from build123d import *

# Parameters (mm, degrees)
F1_DEPTH = 25.4
F2_T     = -0.254


with BuildPart() as f1:
    # F0 (on Top) → F1 (new body)
    with BuildSketch(Plane.XY):
        with BuildLine():
            Line((-3.175, 0), (0, 0))
            Line((0, 0), (0, 25.4))
            ThreePointArc((0, 25.4), (25.4, 50.8), (50.8, 25.4))
            Line((50.8, 25.4), (50.8, 0))
            Line((50.8, 0), (53.975, 0))
            Line((53.975, 0), (53.975, 25.4))
            ThreePointArc((53.975, 25.4), (25.4, 53.975), (-3.175, 25.4))
            Line((-3.175, 25.4), (-3.175, 0))
        make_face()
    extrude(amount=F1_DEPTH)

    # F2
    f2_openings = [f1.faces().sort_by_distance(p)[0] for p in [
        (-1.5875, 0, 12.7),
    ]]
    offset(amount=F2_T, openings=f2_openings)


solid = f1.part
Here's how the part is built. I have some questions about the finished solid (model axes, mm). A direction names the side the tool comes from. Coordinates: 2 decimals unless noted, no trailing zeros. Write each loop counter-clockwise with the first axis right and the second up, starting at its lowest first coordinate (ties: lowest second). Pieces come first, ordered by that corner, then holes. Notation, with made-up numbers: (16, -37) - (21, -37) arc R21 cw to (21, -32) - close; hole circle Ø2 at (83, 64). An arc over 180 degrees is marked (long way). Use one line per item in the form item = value.
1) I'm going to push flat-ended pins straight in: P1, Ø1.3, axis at x = 52, z = 15, coming from the +Y side; P2, Ø4, axis at x = 28, z = 16, coming from the +Y side; P3, Ø10, axis at x = 39.5, z = 8, coming from the +Y side. Where does each tip first touch, or does it pass through?
Solved:
P1 = 37.36
P2 = 53.97
P3 = 52.49
2) Suppose I cut it at C-C, the plane z = 11. Write out the boundary of the cut face in (x, y) (3 decimals).
Solved:
outline = (-3.175, 0) - (-2.921, 0) - (-2.921, 25.4) arc R28.321 cw to (53.721, 25.4) - (53.721, 0.254) - (51.054, 0.254) - (51.054, 25.4) arc R25.654 ccw to (-0.254, 25.4) - (-0.254, 0) - (0, 0) - (0, 25.4) arc R25.4 cw to (50.8, 25.4) - (50.8, 0) - (53.975, 0) - (53.975, 25.4) arc R28.575 ccw to (-3.175, 25.4) - close
3) Suppose I cut it at B-B, the plane x = 25.4. Write out the boundary of the cut face in (y, z) (3 decimals), plus the area to 3 significant figures.
Solved:
outline = (50.8, 0) - (53.975, 0) - (53.975, 25.4) - (50.8, 25.4) - close; hole (51.054, 0.254) - (53.721, 0.254) - (53.721, 25.146) - (51.054, 25.146) - close
area = 14.3 mm2
4) Thinking about a two-plate mould opening in Y: for faces 6 (the flat face through (51.054, 13, 13)), 7 (the cylindrical face through (24.841, 50.794, 12.522)), 8 (the flat face through (15, 49, 25.4)), 9 (the cylindrical face through (26.03, 53.97, 12.52)), which applies, released by +Y, released by -Y, zero draft, split by the parting line, or undercut?
Solved:
face_6 = undercut
face_7 = released by -Y
face_8 = zero draft
face_9 = released by +Y
5) Suppose I cut it at D-D, the plane x = 33. Write out the boundary of the cut face in (y, z), plus the area to 3 significant figures.
Solved:
outline = (49.64, 0) - (52.95, 0) - (52.95, 25.4) - (49.64, 25.4) - close; hole (49.9, 0.25) - (52.68, 0.25) - (52.68, 25.15) - (49.9, 25.15) - close
area = 14.9 mm2
6) Suppose I cut it at A-A, the plane y = 12. Write out the boundary of the cut face in (x, z) (3 decimals).
Solved:
outline = (-3.175, 0) - (0, 0) - (0, 25.4) - (-3.175, 25.4) - close; (50.8, 0) - (53.975, 0) - (53.975, 25.4) - (50.8, 25.4) - close; hole (-2.921, 0.254) - (-0.254, 0.254) - (-0.254, 25.146) - (-2.921, 25.146) - close; hole (51.054, 0.254) - (53.721, 0.254) - (53.721, 25.146) - (51.054, 25.146) - close
7) On a 3-axis mill with a long thin cutter (end or side, diameter ignored), from which of +Z, -Z, +X, -X, +Y, -Y can I reach the whole of each face in a straight line? I mean faces 1 (the flat face through (53.975, 13, 13)), 2 (the flat face through (-0.254, 13, 13)), 3 (the flat face through (50.8, 13, 13)), 4 (the flat face through (52, 0, 13)), 5 (the cylindrical face through (24.836, 51.048, 12.526)). Say none if no direction works.
Solved:
face_1 = +Z, -Z, +X, +Y, -Y
face_2 = -Y
face_3 = +Z, -Z, -Y
face_4 = +Z, -Z, +X, -X, -Y
face_5 = none
8) I need wall thicknesses on line 1 (X direction, y = 10, z = 8) (3 decimals); line 2 (X direction, y = 30.5, z = 4.75); line 3 (Y direction, x = 44, z = 5.25). Which ranges of each line are inside material? Lowest first, please.
Solved:
line_1 = -3.175 to -2.921, -0.254 to 0, 50.8 to 51.054, 53.721 to 53.975
line_2 = -2.72 to -2.46, 0.26 to 0.52, 50.28 to 50.54, 53.26 to 53.52
line_3 = 42.7 to 43.07, 46.76 to 47.09
